Read the model definition and answer for the solid it produces. Units are mm, in the model's axes. A direction names the side the tool comes from. Coordinates: 2 decimals unless noted, no trailing zeros. Order: outer loops, then holes, each group sorted by start corner. A loop starts at its lowest first (then second) coordinate and runs counter-clockwise, first axis right, second up. Notation, with made-up numbers: (27.25, 11) - (58.25, 11) arc R37 ccw to (58.25, 47) - close; hole circle Ø7 at (-13, -32.75). An arc over 180 degrees is marked (long way). Answer as a JSON object with one key per item and string values. Group by question number.
from build123d import *

# Parameters (mm, degrees)
BOSS_EXTRUDE1_DEPTH = 3
SKETCH2_W           = 21
SKETCH2_H           = 3
CUT_EXTRUDE1_DEPTH  = 3


with BuildPart() as part:
    # Sketch1 → Boss-Extrude1 (new body)
    with BuildSketch(Plane.XY):
        Polygon((-35, 38), (-17.5, 38), (17.5, 38), (35, 38), (35, 20.5), (38, 20.5), (38, -20.5), (35, -20.5), (35, -38), (35, -41), (17.5, -41), (17.5, -38), (-17.5, -38), (-17.5, -41), (-35, -41), (-38, -41), (-38, -38), (-38, -20.5), (-35, -20.5), (-35, 20.5), (-38, 20.5), (-38, 38), align=None)
    extrude(amount=BOSS_EXTRUDE1_DEPTH)

    # Sketch2 → Cut-Extrude1 (cut)
    with BuildSketch(Plane.XY.offset(3)):
        Rectangle(SKETCH2_W, SKETCH2_H)
    extrude(amount=-CUT_EXTRUDE1_DEPTH, mode=Mode.SUBTRACT)


solid = part.part
1. Given pin 1 (0.9 mm diameter, centred on x = 36, z = 1, fed in from -Y); pin 2 (1.5 mm diameter, centred on y = -39.5, z = 1, fed in from +X); pin 3 (1.5 mm diameter, centred on x = 37, z = 1, fed in from +Y), each flat-ended and moving along its own axis, determine where each tip first touches the part or whether it passes through.
2. Straight lines are drawn through the part: L1, parallel to Y at x = -5, z = 1.45; L2, parallel to X at y = -37, z = 1.05; L3, parallel to Y at x = 14.5, z = 1.2. For each, find the intervals that lie inside material, in ascending order.
3. For faces 5 (the flat face through (36, 20.5, 1)), 6 (the flat face through (17.5, -40, 1)), 7 (the flat face through (0, 1.5, 2)), 8 (the flat face through (-37, -20.5, 1)), 9 (the flat face through (35, -31, 1)), determine the directions among +Z, -Z, +X, -X, +Y, -Y from which every point of the face is accessible in a straight line to the end or side of a thin tool.
4. A cutting plane is placed at A-A on z = 1.05. Write down the section's boundary in (x, y), and give its area (3 significant figures).
5. For a pull along X with two mould halves and no side action, classify faces 1 (the flat face through (-17.5, -39, 1)), 2 (the flat face through (35, 29, 1)), 3 (the flat face through (26, -41, 1)), 4 (the flat face through (-35, 0, 1)) as pulls with the +X half, pulls with the -X half, needs draft (parallel to the pull), parting line crosses it, or undercut.
6. A cutting plane is placed at C-C on y = 8.5. Write down the section's boundary in (x, z), and give its area (3 significant figures).
7. A cutting plane is placed at B-B on x = -8. Write down the section's boundary in (y, z), and give its area (3 significant figures).
Derived:
{
 "1": {"pin 1": "stops at y = -20.5", "pin 2": "stops at x = 35", "pin 3": "stops at y = 20.5"},
 "2": {"L1": "y = -38 to -1.5, 1.5 to 38", "L2": "x = -38 to 35", "L3": "y = -38 to 38"},
 "3": {"face 5": "+Z, -Z, +X, +Y", "face 6": "+Z, -Z, -Y", "face 7": "+Z, -Z", "face 8": "+Z, -Z, -X", "face 9": "+Z, -Z, +X, -Y"},
 "4": {"outline": "(-38, -41) - (-17.5, -41) - (-17.5, -38) - (17.5, -38) - (17.5, -41) - (35, -41) - (35, -20.5) - (38, -20.5) - (38, 20.5) - (35, 20.5) - (35, 38) - (-38, 38) - (-38, 20.5) - (-35, 20.5) - (-35, -20.5) - (-38, -20.5) - close; hole (-10.5, -1.5) - (10.5, -1.5) - (10.5, 1.5) - (-10.5, 1.5) - close", "area": "5,600 mm2"},
 "5": {"face 1": "undercut", "face 2": "pulls with the +X half", "face 3": "needs draft", "face 4": "pulls with the -X half"},
 "6": {"outline": "(-35, 0) - (38, 0) - (38, 3) - (-35, 3) - close", "area": "219 mm2"},
 "7": {"outline": "(-38, 0) - (-1.5, 0) - (-1.5, 3) - (-38, 3) - close; (1.5, 0) - (38, 0) - (38, 3) - (1.5, 3) - close", "area": "219 mm2"}
}
